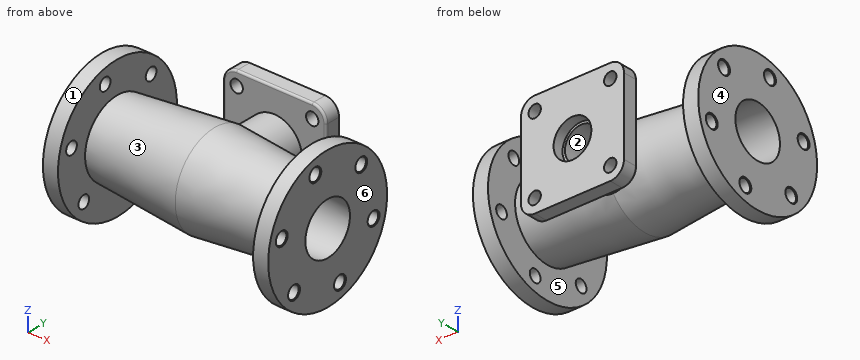
```python
from build123d import *

# Parameters (mm, degrees)
SKETCH6_R                        = 40
SKETCH6_R_2                      = 9
BOSS_EXTRUDE2_DEPTH              = 22
BOSS_EXTRUDE3_REACH              = 295.564
SKETCH6_2_R                      = 40
FILLET1_R                        = 3
F_20_0MM_DOWEL_HOLE2_D           = 18
F_20_0MM_DOWEL_HOLE2_DEPTH       = 22
F_20_0MM_DOWEL_HOLE2_CSINK_D     = 20.05
F_20_0MM_DOWEL_HOLE2_CSINK_ANGLE = 90
CIRPATTERN5_COUNT                = 6
MIRROR1_COPY_1_D                 = 18
MIRROR1_COPY_1_DEPTH             = 22
MIRROR1_COPY_1_CSINK_D           = 20.05
MIRROR1_COPY_1_CSINK_ANGLE       = 90
MIRROR1_COPY_2_D                 = 18
MIRROR1_COPY_2_DEPTH             = 22
MIRROR1_COPY_2_CSINK_D           = 20.05
MIRROR1_COPY_2_CSINK_ANGLE       = 90
MIRROR1_COPY_3_D                 = 18
MIRROR1_COPY_3_DEPTH             = 22
MIRROR1_COPY_3_CSINK_D           = 20.05
MIRROR1_COPY_3_CSINK_ANGLE       = 90
MIRROR1_COPY_4_D                 = 18
MIRROR1_COPY_4_DEPTH             = 22
MIRROR1_COPY_4_CSINK_D           = 20.05
MIRROR1_COPY_4_CSINK_ANGLE       = 90
MIRROR1_COPY_5_D                 = 18
MIRROR1_COPY_5_DEPTH             = 22
MIRROR1_COPY_5_CSINK_D           = 20.05
MIRROR1_COPY_5_CSINK_ANGLE       = 90


with BuildPart() as part:
    # Sketch1 → Revolve1 (revolve)
    with BuildSketch(Plane.XY, mode=Mode.PRIVATE) as revolve1_sk:
        Polygon((0, -51.848140818), (-164, -37.5), (-164, -100), (-142, -100), (-142, -54.482048161), (0, -66.905438381), (142, -54.482048161), (142, -100), (164, -100), (164, -37.5), align=None)
    revolve(revolve1_sk.sketch.rotate(Axis((0, 0, 0), (-1, 0, 0)), 270), axis=Axis((0, 0, 0), (-1, 0, 0)))

    # Sketch6<2> → Boss-Extrude3 (add, up to next)
    with BuildSketch(Plane(origin=(0, 122, 0), x_dir=(1, 0, 0), z_dir=(0, 1, 0)), mode=Mode.PRIVATE) as boss_extrude3_sk1:
        with Locations(Location((0, 0, 0), (0, 0, 90))):
            Circle(SKETCH6_2_R)
    boss_extrude3_tool1 = extrude(boss_extrude3_sk1.sketch, amount=-BOSS_EXTRUDE3_REACH, mode=Mode.PRIVATE) - part.part


with BuildPart() as body_2:
    # Sketch6 → Boss-Extrude2 (new body)
    with BuildSketch(Plane(origin=(0, 122, 0), x_dir=(1, 0, 0), z_dir=(0, 1, 0))):
        with BuildLine():
            Line((-55, 75), (55, 75))
            ThreePointArc((55, 75), (69.142135624, 69.142135624), (75, 55))
            Line((75, 55), (75, -55))
            ThreePointArc((75, -55), (69.142135624, -69.142135624), (55, -75))
            Line((55, -75), (-55, -75))
            ThreePointArc((-55, -75), (-69.142135624, -69.142135624), (-75, -55))
            Line((-75, -55), (-75, 55))
            ThreePointArc((-75, 55), (-69.142135624, 69.142135624), (-55, 75))
        make_face()
        with Locations(Location((0, 0, 0), (0, 0, 270))):
            Circle(SKETCH6_R, mode=Mode.SUBTRACT)
        with Locations(Location((-55, 55, 0), (0, 0, 270))):
            Circle(SKETCH6_R_2, mode=Mode.SUBTRACT)
        with Locations(Location((-55, -55, 0), (0, 0, 270))):
            Circle(SKETCH6_R_2, mode=Mode.SUBTRACT)
        with Locations(Location((55, -55, 0), (0, 0, 270))):
            Circle(SKETCH6_R_2, mode=Mode.SUBTRACT)
        with Locations(Location((55, 55, 0), (0, 0, 270))):
            Circle(SKETCH6_R_2, mode=Mode.SUBTRACT)
    extrude(amount=-BOSS_EXTRUDE2_DEPTH)


with BuildPart() as part_1:
    add(part.part)

    add(body_2.part)  # Boss-Extrude3 merges body 2
    add(boss_extrude3_tool1.solids().sort_by_distance((0, 122, 0))[0])

    # Sketch8 → Cut-Revolve1 (revolve, cut)
    with BuildSketch(Plane.XY, mode=Mode.PRIVATE) as cut_revolve1_sk:
        Polygon((0, 122), (0, 51.219037993), (23.026339686, 51.219037993), (24, 107), (27.5, 107), (27.5, 122), align=None)
    revolve(cut_revolve1_sk.sketch.rotate(Axis((0, -127.507832113, 0), (0, 1, 0)), 90), axis=Axis((0, -127.507832113, 0), (0, 1, 0)), mode=Mode.SUBTRACT)

    # Fillet1
    fillet1_edges = [part_1.edges().sort_by_distance(p)[0] for p in [
        (69.142135624, 100, -69.142135624),
        (75, 100, 0),
        (69.142135624, 100, 69.142135624),
        (0, 100, 75),
        (-69.142135624, 100, 69.142135624),
        (-75, 100, 0),
        (-69.142135624, 100, -69.142135624),
        (0, 100, -75),
    ]]
    fillet(fillet1_edges, radius=FILLET1_R)

    # Ø20.0mm Dowel Hole2
    with Locations(Plane(origin=(164, 0, 0), x_dir=(0, 0, -1), z_dir=(1, 0, 0))):
        with Locations((-77.274066103, -20.705523608)):
            f_20_0mm_dowel_hole2 = CounterSinkHole(F_20_0MM_DOWEL_HOLE2_D / 2, F_20_0MM_DOWEL_HOLE2_CSINK_D / 2, depth=F_20_0MM_DOWEL_HOLE2_DEPTH, counter_sink_angle=F_20_0MM_DOWEL_HOLE2_CSINK_ANGLE)

    # CirPattern5: Ø20.0mm Dowel Hole2 ×6 about axis
    cirpattern5_axis = Axis((0, 0, 0), (1, 0, 0))
    for i in range(1, CIRPATTERN5_COUNT):
        add(f_20_0mm_dowel_hole2.rotate(cirpattern5_axis, i * 360 / CIRPATTERN5_COUNT), mode=Mode.SUBTRACT)

    # Mirror1: Ø20.0mm Dowel Hole2 across plane
    add(f_20_0mm_dowel_hole2.mirror(Plane(origin=(0, 0, 0), x_dir=(0, 0, 1), z_dir=(1, 0, 0))), mode=Mode.SUBTRACT)

    # Mirror1 copy 1
    with Locations(Plane(origin=(-164, 0, 0), x_dir=(0, 0.8660254037844386, -0.5000000000000001), z_dir=(-1, 0, 0))):
        with Locations((-77.274066103, 20.705523608)):
            CounterSinkHole(MIRROR1_COPY_1_D / 2, MIRROR1_COPY_1_CSINK_D / 2, depth=MIRROR1_COPY_1_DEPTH, counter_sink_angle=MIRROR1_COPY_1_CSINK_ANGLE)

    # Mirror1 copy 2
    with Locations(Plane(origin=(-164, 0, 0), x_dir=(0, 0.8660254037844387, 0.4999999999999998), z_dir=(-1, 0, 0))):
        with Locations((-77.274066103, 20.705523608)):
            CounterSinkHole(MIRROR1_COPY_2_D / 2, MIRROR1_COPY_2_CSINK_D / 2, depth=MIRROR1_COPY_2_DEPTH, counter_sink_angle=MIRROR1_COPY_2_CSINK_ANGLE)

    # Mirror1 copy 3
    with Locations(Plane.ZY.offset(164)):
        with Locations((-77.274066103, 20.705523608)):
            CounterSinkHole(MIRROR1_COPY_3_D / 2, MIRROR1_COPY_3_CSINK_D / 2, depth=MIRROR1_COPY_3_DEPTH, counter_sink_angle=MIRROR1_COPY_3_CSINK_ANGLE)

    # Mirror1 copy 4
    with Locations(Plane(origin=(-164, 0, 0), x_dir=(0, -0.8660254037844384, 0.5000000000000004), z_dir=(-1, 0, 0))):
        with Locations((-77.274066103, 20.705523608)):
            CounterSinkHole(MIRROR1_COPY_4_D / 2, MIRROR1_COPY_4_CSINK_D / 2, depth=MIRROR1_COPY_4_DEPTH, counter_sink_angle=MIRROR1_COPY_4_CSINK_ANGLE)

    # Mirror1 copy 5
    with Locations(Plane(origin=(-164, 0, 0), x_dir=(0, -0.8660254037844386, -0.5000000000000001), z_dir=(-1, 0, 0))):
        with Locations((-77.274066103, 20.705523608)):
            CounterSinkHole(MIRROR1_COPY_5_D / 2, MIRROR1_COPY_5_CSINK_D / 2, depth=MIRROR1_COPY_5_DEPTH, counter_sink_angle=MIRROR1_COPY_5_CSINK_ANGLE)


solid = part_1.part
```
The listing builds one solid part. Answer for the finished solid, in the listing's coordinates (mm). Face numbers are marked on the shaded views. A direction names the side the tool comes from. Coordinates: 2 decimals unless noted, no trailing zeros. Write each loop counter-clockwise with the first axis right and the second up, starting at its lowest first coordinate (ties: lowest second). Pieces come first, ordered by that corner, then holes.
Q1. Section B-B, the plane y = 0 is taken. Write down the section's boundary in (x, z), then the cut area to 3 significant figures.
Returned:
outline: (-164, -100) - (-142, -100) - (-142, -54.48) - (0, -66.91) - (142, -54.48) - (142, -100) - (164, -100) - (164, -37.5) - (0, -51.85) - (-164, -37.5) - close; (-164, 37.5) - (0, 51.85) - (164, 37.5) - (164, 100) - (142, 100) - (142, 54.48) - (0, 66.91) - (-142, 54.48) - (-142, 100) - (-164, 100) - close
area: 14,000 mm2
Q2. Find the intervals of material crossed by line 1 along X through (y, z) = (108.5, -55); line 2 along X through (y, z) = (117, 0); line 3 along X through (y, z) = (-57.5, 40), in increasing order.
Returned:
line 1: x = -75 to -64, -46 to 46, 64 to 75
line 2: x = -75 to -27.5, 27.5 to 75
line 3: x = -164 to -142, 142 to 164
Q3. Given P1, Ø20.5, axis at x = 55, z = 55, coming from the -Y side; P2, Ø4, axis at x = -37, z = 74.5, coming from the -Y side; P3, Ø21, axis at x = 21.5, y = 110, coming from the -Z side; P4, Ø14.5, axis at y = 20.71, z = -77.27, coming from the +X side, each flat-ended and moving along its own axis, determine where each tip first touches the part or whether it passes through.
Returned:
P1: stops at y = -43.13
P2: stops at y = 100.04
P3: stops at z = -75
P4: passes through
Q4. The mould has two halves that part along Y. Classify the marked faces 1, 2, 3 and 4: released by +Y, released by -Y, zero draft, split by the parting line, or undercut.
Returned:
face 1: split by the parting line
face 2: released by +Y
face 3: undercut
face 4: zero draft
Q5. Which of the six approach directions +Z, -Z, +X, -X, +Y, -Y give full straight-line access (tool end or side, diameter ignored) to the marked faces 5 and 6?
Returned:
face 5: none
face 6: +Z, -Z, +X, +Y, -Y
Q6. Section A-A, the plane x = 68 is taken. Give the number of separate pieces and of enclosed holes in the cut face, then the cut area to 3 significant figures.
Returned:
separate pieces: 2
enclosed holes: 1
area: 8,140 mm2
